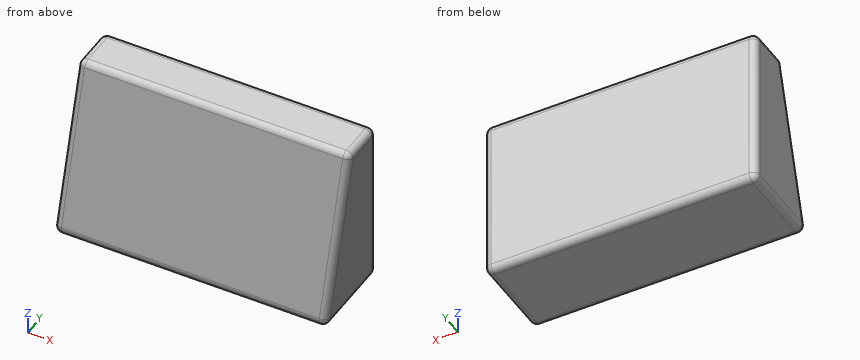
from build123d import *

# Parameters (mm, degrees)
F0_W     = 755.65
F0_H     = 254
F1_DEPTH = 457.2
F3_DEPTH = 755.651
F4_R     = 19.05


with BuildPart() as f1:
    # F0 (on Top) → F1 (new body)
    with BuildSketch(Plane.XY):
        Rectangle(F0_W, F0_H)
    extrude(amount=F1_DEPTH)

    # F2 (on face) → F3 (cut, through all)
    with BuildSketch(Plane.YZ.offset(377.825)):
        Polygon((-127, 457.2), (-127, 0), (0, 457.2), align=None)
    extrude(amount=-F3_DEPTH, mode=Mode.SUBTRACT)

    # F4
    f4_edges = [f1.edges().sort_by_distance(p)[0] for p in [
        (0, -127, 0),
        (377.825, 0, 0),
        (377.825, -63.5, 228.6),
        (-377.825, -63.5, 228.6),
        (-377.825, 0, 0),
        (-377.825, 63.5, 457.2),
        (0, 0, 457.2),
        (377.825, 63.5, 457.2),
        (377.825, 127, 228.6),
        (0, 127, 0),
        (-377.825, 127, 228.6),
        (0, 127, 457.2),
    ]]
    fillet(f4_edges, radius=F4_R)


solid = f1.part
Build history of the part. All positions in model axes, mm. Round coordinates to 2 decimals unless told otherwise and drop trailing zeros. Loops run counter-clockwise (first coordinate to the right, second up) from the corner with the lowest first, then second, coordinate; pieces in that order, holes last. Notation, with made-up numbers: (33, -30) -> (78, -30) arc R17 cw to (78, -26) -> close; hole circle Ø10 at (39.5, 74.25). An arc over 180 degrees is marked (long way). Answer in a Markdown table with one row per item.
Item 1: Saw through at A-A (x = 67). Write the cut outline in (y, z).
Answers below:
| item | result |
|---|---|
| outline | (-120.29, 24.15) arc R19.05 ccw to (-101.94, 0) -> (107.95, 0) arc R19.05 ccw to (127, 19.05) -> (127, 438.15) arc R19.05 ccw to (107.95, 457.2) -> (14.48, 457.2) arc R19.05 ccw to (-3.88, 443.25) -> close |
Item 2: Pin check, flat tip, straight feed: pin 1 (4 mm diameter, centred on x = 6.5, z = 49.5, fed in from -Y). Stop position of the tip, or through.
Answers below:
| item | result |
|---|---|
| pin 1 | stops at y = -113.81 |
Item 3: Drill centre lines: L1, parallel to X at y = -48.5, z = 219; L2, parallel to Y at x = 124, z = 175.5; L3, parallel to Z at x = -148.5, y = 10.5. Where is each one in solid material? Low to high. Write a range as [from, to].
Answers below:
| item | result |
|---|---|
| L1 | x = [-377.72, 377.72] |
| L2 | y = [-78.25, 127] |
| L3 | z = [0, 456.78] |
